Source: CAD feature listing. Evaluate the final solid. Frame: model axes, mm. Face numbers are marked on the shaded views. A direction names the side the tool comes from. Give positions to 0.01 mm unless a question says otherwise; leave off trailing zeros. Loops run counter-clockwise (first coordinate to the right, second up) from the corner with the lowest first, then second, coordinate; pieces in that order, holes last. Notation, with made-up numbers: (81, -36.75) - (95, -36.75) arc R17 cw to (95, -25.75) - close; hole circle Ø4 at (38, 84). An arc over 180 degrees is marked (long way). Put each result on its own line as item: value.
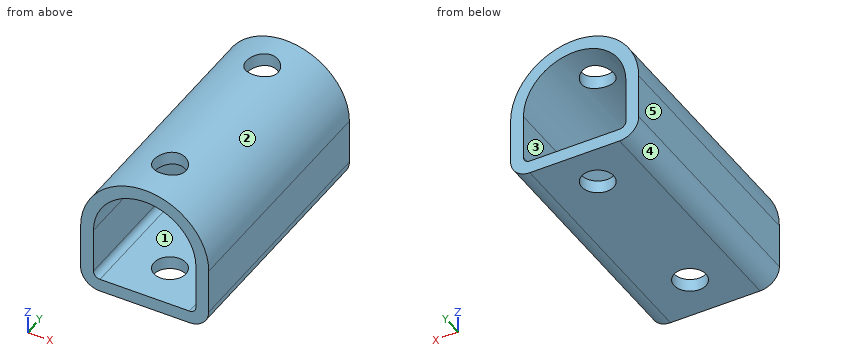
```python
from build123d import *

# Parameters (mm, degrees)
F1_DEPTH      = 76.2
F2_R          = 4.99999
F3_DEPTH      = 20.00096
F3_DEPTH_BACK = 25.4


with BuildPart() as f1:
    # F0 (on Front) → F1 (new body)
    with BuildSketch(Plane.XZ):
        with BuildLine():
            ThreePointArc((19.99996, 0), (0, 19.99996), (-19.99996, 0))
            Line((-19.99996, 0), (-19.99996, -14.00556))
            ThreePointArc((-19.99996, -14.00556), (-18.2442408891, -18.2442408891), (-14.00556, -19.99996))
            Line((-14.00556, -19.99996), (14.00556, -19.99996))
            ThreePointArc((14.00556, -19.99996), (18.2442408891, -18.2442408891), (19.99996, -14.00556))
            Line((19.99996, -14.00556), (19.99996, 0))
        make_face()
        with BuildLine():
            Line((-15.99946, -13.96746), (-15.99946, 0))
            ThreePointArc((-15.99946, 0), (0, 15.99946), (15.99946, 0))
            Line((15.99946, 0), (15.99946, -13.96746))
            ThreePointArc((15.99946, -13.96746), (15.4043009794, -15.4043009794), (13.96746, -15.99946))
            Line((13.96746, -15.99946), (-13.96746, -15.99946))
            ThreePointArc((-13.96746, -15.99946), (-15.4043009794, -15.4043009794), (-15.99946, -13.96746))
        make_face(mode=Mode.SUBTRACT)
    extrude(amount=F1_DEPTH)

    # F2 (on Top) → F3 (cut, two sides)
    with BuildSketch(Plane.XY) as f3_sk:
        with Locations((0, -62.4967)):
            Circle(F2_R)
        with Locations((0, -12.4968)):
            Circle(F2_R)
    extrude(amount=-F3_DEPTH, mode=Mode.SUBTRACT)
    extrude(f3_sk.sketch, amount=F3_DEPTH_BACK, mode=Mode.SUBTRACT)


solid = f1.part
```
1) Pin query (flat end, axial travel): P1, Ø1, axis at y = -11.5, z = 13, coming from the -X side; P2, Ø3, axis at x = -6, y = -21.5, coming from the +Z side; P3, Ø6, axis at y = -40, z = 10, coming from the +X side. Return the tip coordinate at first contact, or that it passes through.
Check result:
P1: x = -15.61
P2: z = 19.49
P3: x = 18.73
2) Section query A-A, the plane z = -7.5. Output: boundary loops of the cut face in (x, y).
Check result:
outline: (-20, -76.2) - (-16, -76.2) - (-16, 0) - (-20, 0) - close; (16, -76.2) - (20, -76.2) - (20, 0) - (16, 0) - close
3) Mould query, pull axis Z, two halves, no side actions, for the marked faces 3, 4 and 5. Classes: pulls with the +Z half, pulls with the -Z half, needs draft (parallel to the pull), parting line crosses it, or undercut.
Check result:
face 3: undercut
face 4: pulls with the -Z half
face 5: needs draft
4) Section query D-D, the plane x = 8.5. Output: boundary loops of the cut face in (y, z).
Check result:
outline: (-76.2, -20) - (0, -20) - (0, -16) - (-76.2, -16) - close; (-76.2, 13.55) - (0, 13.55) - (0, 18.1) - (-76.2, 18.1) - close
5) Access query for the marked faces 1 and 2. Directions: +Z, -Z, +X, -X, +Y, -Y. A direction counts if a zero-diameter tool reaches every point of the face in a straight line with its end or side. Return the directions, or none.
Check result:
face 1: +Y, -Y
face 2: +Z, +Y, -Y
6) Material intervals for line 1 along Y through (x, z) = (0, 17); line 2 along X through (y, z) = (-13, -2); line 3 along Z through (x, y) = (0.5, -54), sorted ascending. Write a range as [from, to].
Check result:
line 1: [-76.2, -67.5], [-57.5, -17.5], [-7.5, 0]
line 2: [-20, -16], [16, 20]
line 3: [-20, -16], [15.99, 19.99]
7) Section query B-B, the plane y = -23. Output: boundary loops of the cut face in (x, z), plus the area to 3 significant figures.
Check result:
outline: (-20, -14.01) arc R5.99 ccw to (-14.01, -20) - (14.01, -20) arc R5.99 ccw to (20, -14.01) - (20, 0) arc R20 ccw to (-20, 0) - close; hole (-16, -13.97) arc R2.03 ccw to (-13.97, -16) - (13.97, -16) arc R2.03 ccw to (16, -13.97) - (16, 0) arc R16 ccw to (-16, 0) - close
area: 501 mm²
8) Section query C-C, the plane x = 0. Output: boundary loops of the cut face in (y, z), plus the area to 3 significant figures.
Check result:
outline: (-76.2, -20) - (-67.5, -20) - (-67.5, -16) - (-76.2, -16) - close; (-76.2, 16) - (-67.5, 16) - (-67.5, 20) - (-76.2, 20) - close; (-57.5, -20) - (-17.5, -20) - (-17.5, -16) - (-57.5, -16) - close; (-57.5, 16) - (-17.5, 16) - (-17.5, 20) - (-57.5, 20) - close; (-7.5, -20) - (0, -20) - (0, -16) - (-7.5, -16) - close; (-7.5, 16) - (0, 16) - (0, 20) - (-7.5, 20) - close
area: 450 mm²
